Input: part model. Units: mm. Frame: model coordinates. Face numbers are marked on the shaded views. A direction names the side the tool comes from. Give positions to 0.01 mm unless a question says otherwise; leave off trailing zeros. Loops run counter-clockwise (first coordinate to the right, second up) from the corner with the lowest first, then second, coordinate; pieces in that order, holes last. Notation, with made-up numbers: (-20, -12) - (13, -12) arc R15 ccw to (13, 6) - close; hole circle Ø11 at (29.25, 11.25). An arc over 180 degrees is marked (long way). One line per item, written item: value.
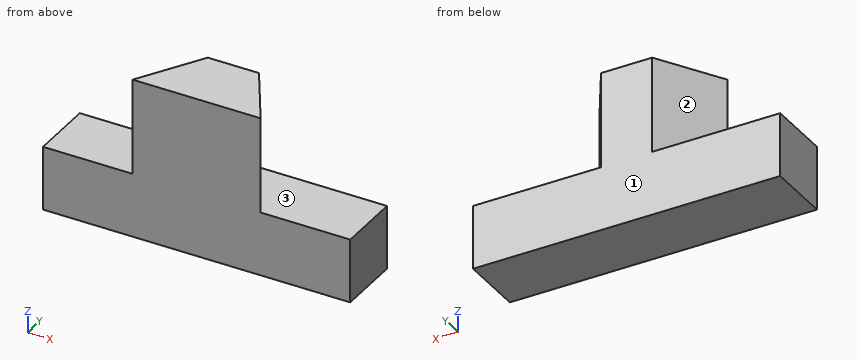
from build123d import *

# Parameters (mm, degrees)
F0_W     = 48
F0_H     = 25
F1_DEPTH = 10
F3_DEPTH = 15


with BuildPart() as f1:
    # F0 (on Front) → F1 (new body)
    with BuildSketch(Plane.XZ):
        Rectangle(F0_W, F0_H)
    extrude(amount=-F1_DEPTH)

    # F2 (on face) → F3 (cut)
    with BuildSketch(Plane.XY.offset(12.5)):
        Polygon((-24, 0), (-10, 0), (-4, 10), (-24, 10), align=None)
        Polygon((4, 10), (10, 0), (24, 0), (24, 10), align=None)
    extrude(amount=-F3_DEPTH, mode=Mode.SUBTRACT)


solid = f1.part
Item 1: Section A-A, the plane y = 8.5. Output: boundary loops of the cut face in (x, z).
Verdict:
outline: (-24, -12.5) - (24, -12.5) - (24, -2.5) - (4.9, -2.5) - (4.9, 12.5) - (-4.9, 12.5) - (-4.9, -2.5) - (-24, -2.5) - close
Item 2: Section B-B, the plane x = -4.5. Output: boundary loops of the cut face in (y, z).
Verdict:
outline: (0, -12.5) - (10, -12.5) - (10, -2.5) - (9.17, -2.5) - (9.17, 12.5) - (0, 12.5) - close
Item 3: Section C-C, the plane y = 1. Output: boundary loops of the cut face in (x, z), and give its area (3 significant figures).
Verdict:
outline: (-24, -12.5) - (24, -12.5) - (24, -2.5) - (9.4, -2.5) - (9.4, 12.5) - (-9.4, 12.5) - (-9.4, -2.5) - (-24, -2.5) - close
area: 762 mm^2
Item 4: Access query for the marked faces 1, 2 and 3. Directions: +Z, -Z, +X, -X, +Y, -Y. A direction counts if a zero-diameter tool reaches every point of the face in a straight line with its end or side. Return the directions, or none.
Verdict:
face 1: +Z, -Z, +X, -X, +Y
face 2: +Z, -X, +Y
face 3: +Z, +X, +Y
Item 5: Material intervals for L1, parallel to Z at x = -10, y = 1.25; L2, parallel to X at y = 2.5, z = 5; L3, parallel to X at y = 4.25, z = 10.25, sorted ascending.
Verdict:
L1: z = -12.5 to -2.5
L2: x = -8.5 to 8.5
L3: x = -7.45 to 7.45
Item 6: Section D-D, the plane z = 9.25. Output: boundary loops of the cut face in (x, y), and give its area (3 significant figures).
Verdict:
outline: (-10, 0) - (10, 0) - (4, 10) - (-4, 10) - close
area: 140 mm^2
Item 7: Pin query (flat end, axial travel): P1, Ø12, axis at x = 10, z = 7, coming from the -Y side; P2, Ø3, axis at x = -14, y = 3, coming from the +Z side. Return the tip coordinate at first contact, or that it passes through.
Verdict:
P1: stops at y = 0
P2: stops at z = -2.5
